from build123d import *

# Parameters (mm, degrees)
SKETCH1_W           = 5.2
SKETCH1_H           = 12
BOSS_EXTRUDE1_DEPTH = 5


with BuildPart() as part:
    # Sketch1 → Boss-Extrude1 (new body)
    with BuildSketch(Plane(origin=(0, 0, 0), x_dir=(1, 0, 0), z_dir=(0, 1, 0))):
        with BuildLine():
            Line((56.6, 26.468421053), (56.6, -33.531578947))
            Line((56.6, -33.531578947), (46.6, -33.531578947))
            Line((46.6, -33.531578947), (46.6, -38.631578947))
            Line((46.6, -38.631578947), (31.6, -38.631578947))
            Line((31.6, -38.631578947), (31.6, -33.531578947))
            Line((31.6, -33.531578947), (28.8, -33.531578947))
            Line((28.8, -33.531578947), (28.8, -18.631578947))
            ThreePointArc((28.8, -18.631578947), (15.8, -5.631578947), (2.8, -18.631578947))
            Line((2.8, -18.631578947), (2.8, -33.531578947))
            Line((2.8, -33.531578947), (0, -33.531578947))
            Line((0, -33.531578947), (0, -38.631578947))
            Line((0, -38.631578947), (-15, -38.631578947))
            Line((-15, -38.631578947), (-15, -33.531578947))
            Line((-15, -33.531578947), (-38.2, -33.531578947))
            Line((-38.2, -33.531578947), (-38.2, -38.631578947))
            Line((-38.2, -38.631578947), (-53.2, -38.631578947))
            Line((-53.2, -38.631578947), (-53.2, -33.531578947))
            Line((-53.2, -33.531578947), (-76.4, -33.531578947))
            Line((-76.4, -33.531578947), (-76.4, -38.631578947))
            Line((-76.4, -38.631578947), (-91.4, -38.631578947))
            Line((-91.4, -38.631578947), (-91.4, -33.531578947))
            Line((-91.4, -33.531578947), (-116.4, -33.531578947))
            Line((-116.4, -33.531578947), (-116.4, 26.468421053))
            Line((-116.4, 26.468421053), (-91.4, 26.468421053))
            Line((-91.4, 26.468421053), (-91.4, 31.568421053))
            Line((-91.4, 31.568421053), (-76.4, 31.568421053))
            Line((-76.4, 31.568421053), (-76.4, 26.468421053))
            Line((-76.4, 26.468421053), (-53.2, 26.468421053))
            Line((-53.2, 26.468421053), (-53.2, 31.568421053))
            Line((-53.2, 31.568421053), (-38.2, 31.568421053))
            Line((-38.2, 31.568421053), (-38.2, 26.468421053))
            Line((-38.2, 26.468421053), (-15, 26.468421053))
            Line((-15, 26.468421053), (-15, 31.568421053))
            Line((-15, 31.568421053), (0, 31.568421053))
            Line((0, 31.568421053), (0, 26.468421053))
            Line((0, 26.468421053), (31.6, 26.468421053))
            Line((31.6, 26.468421053), (31.6, 31.568421053))
            Line((31.6, 31.568421053), (46.6, 31.568421053))
            Line((46.6, 31.568421053), (46.6, 26.468421053))
            Line((46.6, 26.468421053), (56.6, 26.468421053))
        make_face()
        with Locations((51, 8.468421053)):
            Rectangle(SKETCH1_W, SKETCH1_H, mode=Mode.SUBTRACT)
        with Locations((51, -15.531578947)):
            Rectangle(SKETCH1_W, SKETCH1_H, mode=Mode.SUBTRACT)
    extrude(amount=BOSS_EXTRUDE1_DEPTH)


solid = part.part
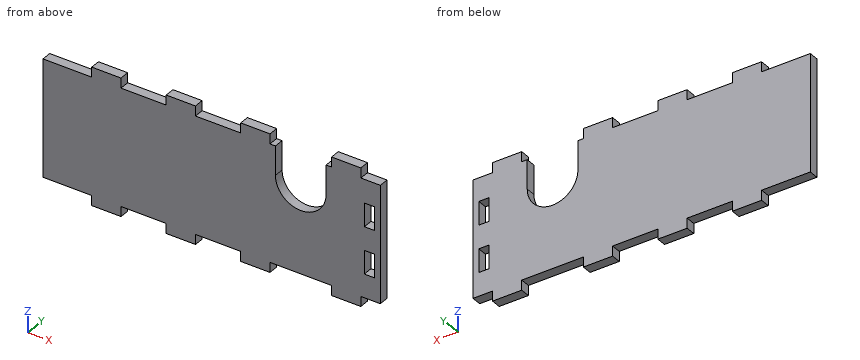
The model under review builds one solid part; all positions refer to its coordinate system, in mm. Coordinates: 2 decimals unless noted, no trailing zeros. Write each loop counter-clockwise with the first axis right and the second up, starting at its lowest first coordinate (ties: lowest second). Pieces come first, ordered by that corner, then holes. Notation, with made-up numbers: (-30, 85.25) - (-13, 85.25) arc R27 cw to (-13, 110.25) - close; hole circle Ø11 at (71, -24). An arc over 180 degrees is marked (long way). Answer as a JSON object with one key per item and string values. Group by question number.
1. Add section A-A (z = -5). Give the boundary of the cut face in (x, y).
2. Add section B-B (y = 4.05). Give the number of separate pieces and of enclosed holes in the cut face, plus the area to 3 significant figures.
3. Add section D-D (x = 15.8). Give the boundary of the cut face in (y, z).
4. Add section C-C (z = 28). Give the boundary of the cut face in (x, y), plus the area to 3 significant figures.
5. To check wall thickness, follow probe 1 along X at (y, z) = (4.55, 36); probe 2 along X at (y, z) = (1.55, 29.5); probe 3 along X at (y, z) = (0.8, 16). State the ranges of each line that lie inside material, in increasing order.
6. Clearance check with flat-ended pins moving along their axes: pin 1 Ø0.8 at (x, y) = (30, 1.5) entering from +Z; pin 2 Ø1.5 at (y, z) = (3.5, 35) entering from +X; pin 3 Ø2.5 at (x, y) = (17.5, 2) entering from -Z. State where each tip first meets the part, or that it passes through.
Findings:
{
 "1": {"outline": "(-116.4, 0) - (48.4, 0) - (48.4, 5) - (-116.4, 5) - close; (53.6, 0) - (56.6, 0) - (56.6, 5) - (53.6, 5) - close"},
 "2": {"separate pieces": "1", "enclosed holes": "2", "area": "10,200 mm²"},
 "3": {"outline": "(0, -26.47) - (5, -26.47) - (5, 5.63) - (0, 5.63) - close"},
 "4": {"outline": "(-116.4, 0) - (2.8, 0) - (2.8, 5) - (-116.4, 5) - close; (28.8, 0) - (56.6, 0) - (56.6, 5) - (28.8, 5) - close", "area": "735 mm²"},
 "5": {"probe 1": "-91.4 to -76.4, -53.2 to -38.2, -15 to 0, 31.6 to 46.6", "probe 2": "-116.4 to 2.8, 28.8 to 56.6", "probe 3": "-116.4 to 3.07, 28.53 to 48.4, 53.6 to 56.6"},
 "6": {"pin 1": "z = 33.53", "pin 2": "x = 46.6", "pin 3": "z = -26.47"}
}
